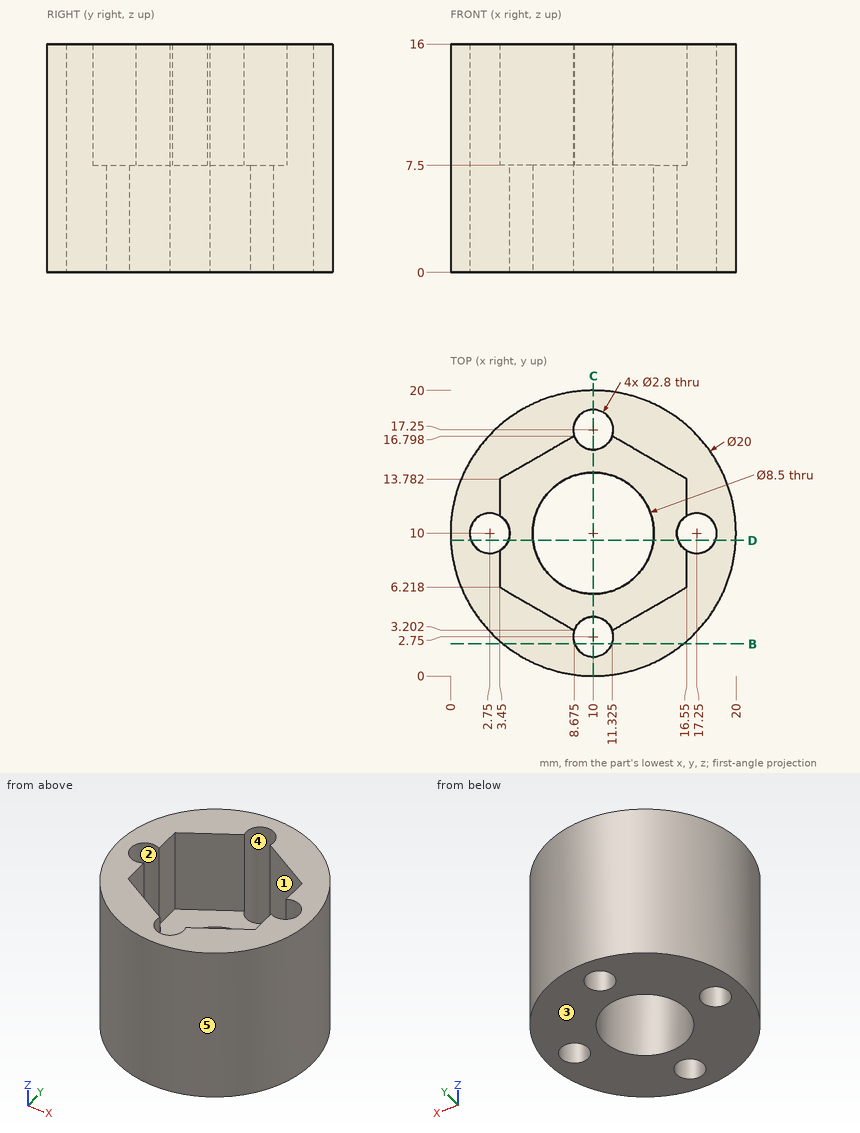
Design review of the part shown in the three views and the two pictorial views. Dimensions are in mm from the part's minimum x, y and z. A direction names the side the tool comes from. Round coordinates to 2 decimals unless told otherwise and drop trailing zeros. Loops run counter-clockwise (first coordinate to the right, second up) from the corner with the lowest first, then second, coordinate; pieces in that order, holes last. Notation, with made-up numbers: (-40, 76) - (9, 76) arc R14 ccw to (9, 89) - close; hole circle Ø9 at (-26, 82). An arc over 180 degrees is marked (long way). Write each question's results on one line, items separated by ' | '. Start each with the question number.
Q1. Take a section at D-D on y = 9.5. Give the boundary of the cut face in (x, z).
Q2. Take a section at B-B on y = 2.25. Give the boundary of the cut face in (x, z).
Q3. Insertion check: P1, Ø2, axis at y = 12, z = 11, coming from the +X side; P2, Ø4, axis at x = 12.5, y = 7, coming from the +Z side; P3, Ø4, axis at x = 16.5, z = 12.5, coming from the -Y side. Each pin has a flat end and moves straight along its axis. Give the tip position at first contact, or say it passes through.
Q4. Tool access review of the marked faces 1 and 2: name each direction out of +Z, -Z, +X, -X, +Y, -Y from which nothing blocks a thin tool from reaching the whole face with its end or side.
Q5. Draft analysis for pull direction X (two halves, no side actions). For the marked faces 3, 4 and 5, state which applies: pulls with the +X half, pulls with the -X half, needs draft (parallel to the pull), parting line crosses it, or undercut.
Q6. Wall thickness on line 1 along Y through (x, z) = (10, 2.75); line 2 along X through (y, z) = (9.5, 5.5); line 3 along Y through (x, z) = (10, 12.5): over which ranges is each line inside the solid? List them lowest first. Write a range as [from, to].
Q7. Take a section at C-C on x = 10. Give the boundary of the cut face in (y, z).
Data:
1) outline: (0.01, 0) - (1.44, 0) - (1.44, 16) - (0.01, 16) - close; (4.06, 0) - (5.78, 0) - (5.78, 7.5) - (4.06, 7.5) - close; (14.22, 0) - (15.94, 0) - (15.94, 7.5) - (14.22, 7.5) - close; (18.56, 0) - (19.99, 0) - (19.99, 16) - (18.56, 16) - close
2) outline: (3.68, 0) - (8.69, 0) - (8.69, 16) - (3.68, 16) - close; (11.31, 0) - (16.32, 0) - (16.32, 16) - (11.31, 16) - close
3) P1: stops at x = 19.95 | P2: stops at z = 7.5 | P3: stops at y = 1.07
4) face 1: +Z | face 2: +Z, -Z
5) face 3: needs draft | face 4: undercut | face 5: parting line crosses it
6) line 1: y = [0, 1.35], [4.15, 5.75], [14.25, 15.85], [18.65, 20] | line 2: x = [0.01, 1.44], [4.06, 5.78], [14.22, 15.94], [18.56, 19.99] | line 3: y = [0, 1.35], [18.65, 20]
7) outline: (0, 0) - (1.35, 0) - (1.35, 16) - (0, 16) - close; (4.15, 0) - (5.75, 0) - (5.75, 7.5) - (4.15, 7.5) - close; (14.25, 0) - (15.85, 0) - (15.85, 7.5) - (14.25, 7.5) - close; (18.65, 0) - (20, 0) - (20, 16) - (18.65, 16) - close
